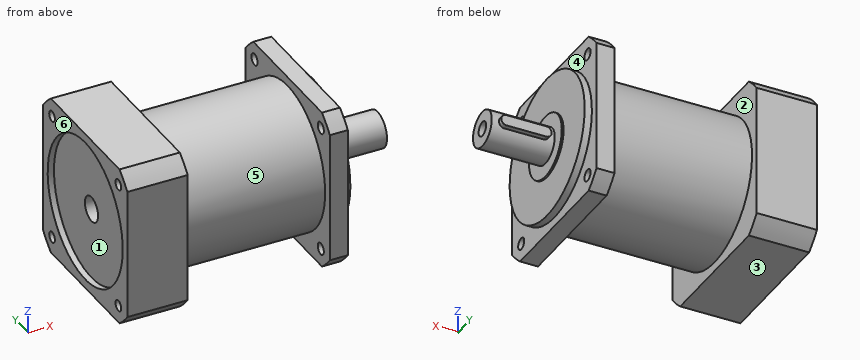
from build123d import *

# Parameters (mm, degrees)
EXTRUDE_1_DEPTH     = 12.5
CUT_EXTRUDE_1_REACH = 71.282
SKETCH_3_R          = 4
SKETCH_4_R          = 3.25
EXTRUDE_2_DEPTH     = 10
SKETCH_5_R          = 40
EXTRUDE_3_DEPTH     = 79
EXTRUDE_4_DEPTH     = 33.5
CUT_EXTRUDE_START   = -3.5
SKETCH_7_R          = 40
CUT_EXTRUDE_2_DEPTH = 3.5
SKETCH_8_R          = 7
CUT_EXTRUDE_3_DEPTH = 30
SKETCH_9_R          = 3
CUT_EXTRUDE_4_DEPTH = 15


with BuildPart() as part:
    # 草图1 → 旋转1 (revolve)
    with BuildSketch(Plane.XY, mode=Mode.PRIVATE) as revolve_1_sk:
        Polygon((0, 0), (0, 40), (4, 40), (4, 17.5), (5, 17.5), (5, 10), (40, 10), (40, 0), align=None)
    revolve(revolve_1_sk.sketch.rotate(Axis((-53.526377828, 0, 0), (1, 0, 0)), 90), axis=Axis((-53.526377828, 0, 0), (1, 0, 0)))

    # 草图2 → 凸台-拉伸1 (add)
    with BuildSketch(Plane(origin=(0, 0, 0), x_dir=(1, 0, 0), z_dir=(0, 1, 0))):
        with BuildLine():
            Line((11, 3), (33, 3))
            ThreePointArc((33, 3), (36, 0), (33, -3))
            Line((33, -3), (11, -3))
            ThreePointArc((11, -3), (8, 0), (11, 3))
        make_face()
    extrude(amount=EXTRUDE_1_DEPTH)

    # 草图3 → 切除-拉伸1 (cut, up to next)
    with BuildSketch(Plane(origin=(40, 0, 0), x_dir=(0, 0, -1), z_dir=(1, 0, 0)), mode=Mode.PRIVATE) as cut_extrude_1_sk1:
        Circle(SKETCH_3_R)
    cut_extrude_1_tool1 = extrude(cut_extrude_1_sk1.sketch, amount=-CUT_EXTRUDE_1_REACH, mode=Mode.PRIVATE) & part.part
    add(cut_extrude_1_tool1.solids().sort_by_distance((40, 0, 0))[0], mode=Mode.SUBTRACT)

    # 草图4 → 凸台-拉伸2 (add)
    with BuildSketch(Plane.ZY):
        with BuildLine():
            Line((36.592348927, -45), (-36.592348927, -45))
            ThreePointArc((-36.592348927, -45), (-41.012193309, -41.012193309), (-45, -36.592348927))
            Line((-45, -36.592348927), (-45, 36.592348927))
            ThreePointArc((-45, 36.592348927), (-41.012193309, 41.012193309), (-36.592348927, 45))
            Line((-36.592348927, 45), (36.592348927, 45))
            ThreePointArc((36.592348927, 45), (41.012193309, 41.012193309), (45, 36.592348927))
            Line((45, 36.592348927), (45, -36.592348927))
            ThreePointArc((45, -36.592348927), (41.012193309, -41.012193309), (36.592348927, -45))
        make_face()
        with Locations((-35.355339059, 35.355339059)):
            Circle(SKETCH_4_R, mode=Mode.SUBTRACT)
        with Locations(Location((35.355339059, -35.355339059, 0), (0, 0, 180))):
            Circle(SKETCH_4_R, mode=Mode.SUBTRACT)
        with Locations((35.355339059, 35.355339059)):
            Circle(SKETCH_4_R, mode=Mode.SUBTRACT)
        with Locations(Location((-35.355339059, -35.355339059, 0), (0, 0, 180))):
            Circle(SKETCH_4_R, mode=Mode.SUBTRACT)
    extrude(amount=EXTRUDE_2_DEPTH)

    # 草图5 → 凸台-拉伸3 (add)
    with BuildSketch(Plane.ZY.offset(10)):
        Circle(SKETCH_5_R)
    extrude(amount=EXTRUDE_3_DEPTH)

    # 草图6 → 凸台-拉伸4 (add)
    with BuildSketch(Plane.ZY.offset(89)):
        with BuildLine():
            Line((36.592348927, 45), (-36.592348927, 45))
            ThreePointArc((-36.592348927, 45), (-41.012193309, 41.012193309), (-45, 36.592348927))
            Line((-45, 36.592348927), (-45, -36.592348927))
            ThreePointArc((-45, -36.592348927), (-41.012193309, -41.012193309), (-36.592348927, -45))
            Line((-36.592348927, -45), (36.592348927, -45))
            ThreePointArc((36.592348927, -45), (41.012193309, -41.012193309), (45, -36.592348927))
            Line((45, -36.592348927), (45, 36.592348927))
            ThreePointArc((45, 36.592348927), (41.012193309, 41.012193309), (36.592348927, 45))
        make_face()
    extrude(amount=EXTRUDE_4_DEPTH)

    # 草图7 → 切除-拉伸2 (cut)
    with BuildSketch(Plane.ZY.offset(122.5).offset(CUT_EXTRUDE_START)):
        Circle(SKETCH_7_R)
    extrude(amount=CUT_EXTRUDE_2_DEPTH, mode=Mode.SUBTRACT)

    # 草图8 → 切除-拉伸3 (cut)
    with BuildSketch(Plane.ZY.offset(122.5)):
        Circle(SKETCH_8_R)
    extrude(amount=-CUT_EXTRUDE_3_DEPTH, mode=Mode.SUBTRACT)

    # 草图9 → 切除-拉伸4 (cut)
    with BuildSketch(Plane.ZY.offset(122.5)):
        with Locations((35.355339059, 35.355339059)):
            Circle(SKETCH_9_R)
        with Locations(Location((-35.355339059, 35.355339059, 0), (0, 0, 180))):
            Circle(SKETCH_9_R)
        with Locations(Location((35.355339059, -35.355339059, 0), (0, 0, 180))):
            Circle(SKETCH_9_R)
        with Locations((-35.355339059, -35.355339059)):
            Circle(SKETCH_9_R)
    extrude(amount=-CUT_EXTRUDE_4_DEPTH, mode=Mode.SUBTRACT)


solid = part.part
Verification items for the finished model (mm, model axes). Face numbers are marked on the shaded views. A direction names the side the tool comes from. Coordinates: 2 decimals unless noted, no trailing zeros. Write each loop counter-clockwise with the first axis right and the second up, starting at its lowest first coordinate (ties: lowest second). Pieces come first, ordered by that corner, then holes. Notation, with made-up numbers: (32.5, -35.75) -> (38.5, -35.75) arc R22 cw to (38.5, -14.75) -> close; hole circle Ø7 at (14.5, 49.5). An arc over 180 degrees is marked (long way). One line per item, written item: value. Start each with the question number.
Q1. Access from +Z, -Z, +X, -X, +Y, -Y to the whole of each face (thin tool, end or side, straight path). Record for the marked faces 4, 5 and 6.
Q2. Thickness scan on L1, parallel to X at y = 41, z = -31.5; L2, parallel to Y at x = -110, z = 0.5; L3, parallel to Y at x = -7, z = -35. Record the ranges inside material, lowest first. Write a range as from..to.
Q3. Go/stop test with flat-tipped pins: P1, Ø9.5, axis at y = 35.36, z = -35.36, coming from the +X side; P2, Ø2, axis at x = -62.5, z = -23.5, coming from the -Y side; P3, Ø12, axis at x = -50, z = 21, coming from the +Y side. Record where each tip stops, or that it passes through.
Q4. Mould release check, pull along Z, two halves, no side actions. Record for the marked faces 1, 2 and 3: pulls with the +Z half, pulls with the -Z half, needs draft (parallel to the pull), parting line crosses it, or undercut.
Q5. Cross-section at A-A on x = -28. Enter the section's corners in (y, z), and give its area (3 significant figures).
Checked values:
1. face 4: +X
1. face 5: none
1. face 6: +Z, -Z, -X, +Y, -Y
2. L1: x = -122.5..-89, -10..0
2. L2: y = -45..-6.98, 6.98..45
2. L3: y = -45..-38.59, -32.12..32.12, 38.59..45
3. P1: stops at x = 0
3. P2: stops at y = -33.07
3. P3: stops at y = 37.08
4. face 1: undercut
4. face 2: needs draft
4. face 3: pulls with the -Z half
5. outline: circle Ø80 at (0, 0)
5. area: 5,030 mm²
